from build123d import *

# Parameters (mm, degrees)
SKETCH1_R           = 9.5
BOSS_EXTRUDE1_DEPTH = 11


with BuildPart() as part:
    # Sketch1 → Boss-Extrude1 (new body)
    with BuildSketch(Plane(origin=(0, 0, 0), x_dir=(1, 0, 0), z_dir=(0, 1, 0))):
        with BuildLine():
            Line((0, 0), (78, 0))
            Line((78, 0), (63.570914871, 40.080792024))
            ThreePointArc((63.570914871, 40.080792024), (58.082802811, 47.272161186), (49.457603693, 50))
            Line((49.457603693, 50), (0, 50))
            Line((0, 50), (0, 0))
        make_face()
        with Locations(Location((39.952273438, 24.5, 0), (0, 0, 270))):
            Circle(SKETCH1_R, mode=Mode.SUBTRACT)
    extrude(amount=BOSS_EXTRUDE1_DEPTH)


solid = part.part
Model file for the job. Use its own axes, mm. Round coordinates to 2 decimals unless told otherwise and drop trailing zeros. Order: outer loops, then holes, each group sorted by start corner. A loop starts at its lowest first (then second) coordinate and runs counter-clockwise, first axis right, second up. Notation, with made-up numbers: M 59.25,8 L 112.25,8 A18 ccw 112.25,42 Z; hole C 55.25,-20 d1. An arc over 180 degrees is marked long. Write each question's results on one line, items separated by ' | '. Start each with the question number.
(1) Saw through at B-B, the plane x = 47. Give the cut face in (y, z).
(2) Saw through at D-D, the plane z = -7. Give the cut face in (x, y), then the cut area to 3 significant figures.
(3) Two-plate mould, pull along X, no slides. Class faces 1 (the face through (70.886, 5.423, -19.76)), 2 (the face through (30.68, 5.42, -26.56)), 3 (the face through (25, 5, -50)): pulls with the +X half, pulls with the -X half, needs draft (parallel to the pull), parting line crosses it, or undercut.
(4) Probe probe 1 along Z at (x, y) = (47.5, 2); probe 2 along X at (y, z) = (7.5, -19); probe 3 along X at (y, z) = (6, -24.5). List the from-to ranges inside material, lowest first. Write a range as from..to.
(5) Drop flat-ended pins along their axis: pin 1 (3 mm diameter, centred on y = 4.5, z = -6, fed in from +X); pin 2 (15 mm diameter, centred on x = 39.95, z = -24.5, fed in from +Y) (3 decimals). Give the stop position or say it passes through.
(6) Saw through at A-A, the plane z = -24.5. Give the cut face in (x, y).
(7) Saw through at C-C, the plane y = 3.25. Give the cut face in (x, z).
Established:
1) outline: M 0,-50 L 11,-50 L 11,-30.87 L 0,-30.87 Z; M 0,-18.13 L 11,-18.13 L 11,0 L 0,0 Z
2) outline: M 0,0 L 75.48,0 L 75.48,11 L 0,11 Z | area: 830 mm^2
3) face 1: pulls with the +X half | face 2: undercut | face 3: needs draft
4) probe 1: z = -50..-30.27, -18.73..0 | probe 2: x = 0..32.21, 47.7..71.16 | probe 3: x = 0..30.45, 49.45..69.18
5) pin 1: stops at x = 76.38 | pin 2: passes through
6) outline: M 0,0 L 30.45,0 L 30.45,11 L 0,11 Z; M 49.45,0 L 69.18,0 L 69.18,11 L 49.45,11 Z
7) outline: M 0,-50 L 49.46,-50 A15 ccw 63.57,-40.08 L 78,0 L 0,0 Z; hole C 39.95,-24.5 d19
